Autodesk Inventor part; units mm, degrees
ref_plane "YZ Plane" through (0, 0, 0) normal (1, 0, 0) x (0, 1, 0)
ref_plane "XZ Plane" through (0, 0, 0) normal (0, 1, 0) x (-1, 0, 0)
ref_plane "XY Plane" through (0, 0, 0) normal (0, 0, 1) x (1, 0, 0)
sketch "Sketch1" plane through (0, 0, 0) normal (0, 1, 0) x (-1, 0, 0)
  line L0 (0, 0) -> (74, 0)
  line L1 (74, 0) -> (74, -74)
  line L2 (74, -74) -> (0, -74)
  line L3 (0, -74) -> (0, 0)
  dimension "d0" = 74
  dimension "d1" = 74
extrude "Extrusion1" add sketch "Sketch1" along normal blind 10
sketch "Sketch2" plane through (0, 10, 0) normal (0, 1, 0) x (1, 0, 0)
  line L0 (0, 0) -> (0, 74)
  line L1 (0, 74) -> (-74, 74)
  line L2 (0, 0) -> (-74, 0)
  line L3 (-74, 0) -> (-74, 74)
  line L4 (-74, 74) -> (0, 74)
  line L5 (0, 74) -> (0, 0)
  line L6 (-72.5, 72.5) -> (-72.5, 1.5)
  line L7 (-72.5, 1.5) -> (-1.5, 1.5)
  line L8 (-1.5, 1.5) -> (-1.5, 72.5)
  line L9 (-1.5, 72.5) -> (-72.5, 72.5)
  dimension "d4" = 1.5
extrude "Extrusion2" add sketch "Sketch2" along normal blind 5
sketch "Sketch3" plane through (0, 0, 0) normal (0, -1, 0) x (1, 0, 0)
  line L0 (0, 0) -> (0, -74)
  line L1 (0, 0) -> (-74, 0)
  line L2 (-74, 0) -> (-74, -74)
  line L3 (-74, -74) -> (0, -74)
  line L4 (0, -74) -> (0, 0)
extrude "Extrusion3" cut sketch "Sketch3" against normal blind 5
properties part number "DiffusorCap"
Verification items for the finished model (mm, model axes). A direction names the side the tool comes from. Coordinates: 2 decimals unless noted, no trailing zeros. Write each loop counter-clockwise with the first axis right and the second up, starting at its lowest first coordinate (ties: lowest second). Pieces come first, ordered by that corner, then holes. Notation, with made-up numbers: M -38.75,-24 L 5.25,-24 A7 ccw 5.25,-19 Z; hole C 81,-20.75 d6. An arc over 180 degrees is marked long. Answer as a JSON object with one key per item and string values. Group by question number.
(1) Gauge pin test, flat end, axial feed: pin 1 (12 mm diameter, centred on x = -55, z = -42, fed in from +Y). Record the tip position at first contact, or that the pin passes through.
(2) Material ranges on line 1 (Z direction, x = -48, y = 12); line 2 (Y direction, x = -39.5, z = -40.5), recorded low to high.
(3) Release check for a two-part mould opening along Z. For faces 1 (the face through (-37, 10, -37)), 2 (the face through (-38, 5, -36)), 3 (the face through (-38, 10, -74)) record: +Z half, -Z half, draft (parallel to the pull), parting line (faces both ways), or undercut.
(4) Cross-section at C-C, the plane x = -21.5. Record the cut outline in (y, z), and give its area (3 significant figures).
(5) Cross-section at A-A, the plane y = 11.75. Record the cut outline in (x, z), and give its area (3 significant figures).
(6) Tool access check on faces 4 (the face through (-37, 12, -1.5)), 5 (the face through (-54, 15, -73)). Record the directions out of +Z, -Z, +X, -X, +Y, -Y that give a thin tool (end or side, any length) a straight path to the whole face; none if there is none.
(7) Cross-section at B-B, the plane z = -45. Record the cut outline in (x, y).
Reply:
{
 "1": {"pin 1": "y = 10"},
 "2": {"line 1": "-74 to -72.5, -1.5 to 0", "line 2": "5 to 10"},
 "3": {"face 1": "undercut", "face 2": "draft", "face 3": "-Z half"},
 "4": {"outline": "M 5,-74 L 15,-74 L 15,-72.5 L 10,-72.5 L 10,-1.5 L 15,-1.5 L 15,0 L 5,0 Z", "area": "385 mm²"},
 "5": {"outline": "M -74,-74 L 0,-74 L 0,0 L -74,0 Z; hole M -72.5,-72.5 L -1.5,-72.5 L -1.5,-1.5 L -72.5,-1.5 Z", "area": "435 mm²"},
 "6": {"face 4": "+Y", "face 5": "+Z, -Z, +X, -X, +Y"},
 "7": {"outline": "M -74,5 L 0,5 L 0,15 L -1.5,15 L -1.5,10 L -72.5,10 L -72.5,15 L -74,15 Z"}
}
